```python
from build123d import *

# Parameters (mm, degrees)
BOSS_EXTRUDE1_DEPTH = 10
CUT_EXTRUDE2_DEPTH  = 10
FILLET1_R           = 1
FILLET2_R           = 1


with BuildPart() as part:
    # Sketch1 → Boss-Extrude1 (new body)
    with BuildSketch(Plane(origin=(0, 0, 0), x_dir=(1, 0, 0), z_dir=(0, 1, 0))):
        with BuildLine():
            Line((-102.94704138, 26.470588235), (-22.94704138, 26.470588235))
            ThreePointArc((-22.94704138, 26.470588235), (-15.875973568, 23.541656047), (-12.94704138, 16.470588235))
            Line((-12.94704138, 16.470588235), (-12.94704138, -28.529411765))
            ThreePointArc((-12.94704138, -28.529411765), (-15.875973568, -35.600479577), (-22.94704138, -38.529411765))
            Line((-22.94704138, -38.529411765), (-102.94704138, -38.529411765))
            ThreePointArc((-102.94704138, -38.529411765), (-110.018109192, -35.600479577), (-112.94704138, -28.529411765))
            Line((-112.94704138, -28.529411765), (-112.94704138, 16.470588235))
            ThreePointArc((-112.94704138, 16.470588235), (-110.018109192, 23.541656047), (-102.94704138, 26.470588235))
        make_face()
    extrude(amount=BOSS_EXTRUDE1_DEPTH)

    # Sketch2 → Cut-Extrude2 (cut)
    with BuildSketch(Plane(origin=(0, 10, 0), x_dir=(1, 0, 0), z_dir=(0, 1, 0))):
        with BuildLine():
            Line((-86.374151264, -1.785526941), (-53.155911565, -1.785526941))
            add(Edge.make_bspline(
                [(-53.155911565, -1.785526941), (-53.129080982, -1.789380086), (-53.1023159, -1.793281348), (-53.075607342, -1.797231207)],
                knots=[0, 0, 0, 0, 0.0009964, 0.0009964, 0.0009964, 0.0009964], degree=3))
            add(Edge.make_bspline(
                [(-53.075607342, -1.797231207), (-51.541485704, -2.316740326), (-45.415602023, -4.422444293), (-33.321239101, -6.01523888), (-45.249562715, -7.639432102), (-51.251453322, -9.678465504), (-52.693570539, -10.167430322)],
                knots=[0, 0, 0, 0, 0.063344572, 0.23684536, 0.40937521, 0.468351292, 0.468351292, 0.468351292, 0.468351292], degree=3))
            add(Edge.make_bspline(
                [(-52.693570539, -10.167430322), (-52.933080229, -10.206733211), (-53.17537239, -10.242094783), (-53.423139068, -10.273296592)],
                knots=[0.31414383, 0.31414383, 0.31414383, 0.31414383, 0.323514461, 0.323514461, 0.323514461, 0.323514461], degree=3))
            Line((-53.423139068, -10.273296592), (-86.374151264, -10.273296592))
            Line((-86.374151264, -10.273296592), (-86.374151264, -1.785526941))
        make_face()
    extrude(amount=-CUT_EXTRUDE2_DEPTH, mode=Mode.SUBTRACT)

    # Fillet1
    fillet1_edges = [part.edges().sort_by_distance(p)[0] for p in [
        (-110.018109192, 10, -23.541656047),
        (-112.94704138, 10, 6.029411765),
        (-110.018109192, 10, 35.600479577),
        (-62.94704138, 10, 38.529411765),
        (-15.875973568, 10, 35.600479577),
        (-12.94704138, 10, 6.029411765),
        (-15.875973568, 10, -23.541656047),
        (-62.94704138, 10, -26.470588235),
    ]]
    fillet(fillet1_edges, radius=FILLET1_R)

    # Fillet2
    fillet2_edges = [part.edges().sort_by_distance(p)[0] for p in [
        (-112.94704138, 0, 6.029411765),
        (-110.018109192, 0, -23.541656047),
        (-62.94704138, 0, -26.470588235),
        (-15.875973568, 0, -23.541656047),
        (-12.94704138, 0, 6.029411765),
        (-15.875973568, 0, 35.600479577),
        (-62.94704138, 0, 38.529411765),
        (-110.018109192, 0, 35.600479577),
    ]]
    fillet(fillet2_edges, radius=FILLET2_R)


solid = part.part
```
Input: part model. Units: mm. Frame: model coordinates. A direction names the side the tool comes from. Give positions to 0.01 mm unless a question says otherwise; leave off trailing zeros. Write each loop counter-clockwise with the first axis right and the second up, starting at its lowest first coordinate (ties: lowest second). Pieces come first, ordered by that corner, then holes. Notation, with made-up numbers: (46, -3.75) - (77, -3.75) arc R24 ccw to (77, 7.25) - close; hole circle Ø3 at (-27.5, 7). An arc over 180 degrees is marked (long way). Write item = value, one per line. Start each with the question number.
1) Material intervals for L1, parallel to Z at x = -81, y = 8; L2, parallel to Z at x = -38.5, y = 7; L3, parallel to X at y = 2.75, z = 36, sorted ascending. Write a range as [from, to].
2) Pin query (flat end, axial travel): pin 1 (12 mm diameter, centred on x = -34, z = 25.5, fed in from -Y). Return the tip coordinate at first contact, or that it passes through.
3) Reachability of faces 1 (the face through (-70, 5, 10.273)), 2 (the face through (-62, 0, -1)) from +Z, -Z, +X, -X, +Y, -Y: full face, straight path, thin tool, end or side. Return the list, or none.
4) Draft query along X for faces 3 (the face through (-62, 10, -1)), 4 (the face through (-12.947, 5, 6)), 5 (the face through (-86.374, 5, 6)). Return one class per face: pulls with the +X half, pulls with the -X half, needs draft (parallel to the pull), parting line crosses it, or undercut.
5) Cut plane A-A (x = -82.5). Return loops of the section in (y, z).
Answers follow:
q1.L1 = [-26.47, 1.79], [10.27, 38.53]
q1.L2 = [-26.47, 5.88], [6.17, 38.53]
q1.L3 = [-109.59, -16.3]
q2.pin_1 = 0
q3.face_1 = +Y, -Y
q3.face_2 = +Z, -Z, +X, -X, -Y
q4.face_3 = needs draft
q4.face_4 = pulls with the +X half
q4.face_5 = undercut
q5.outline = (0, -25.47) arc R1 ccw to (1, -26.47) - (9, -26.47) arc R1 ccw to (10, -25.47) - (10, 1.79) - (0, 1.79) - close; (0, 10.27) - (10, 10.27) - (10, 37.53) arc R1 ccw to (9, 38.53) - (1, 38.53) arc R1 ccw to (0, 37.53) - close
